Autodesk Fusion 360 part; units mm, degrees
sketch "Sketch1" plane through (0, 0, 0) normal (0, 0, 1) x (1, 0, 0)
  line L0 (0, 0) -> (-27, 0)
  line L1 (-27, 0) -> (-27, 4)
  line L2 (-27, 4) -> (-20.5209, 4)
  line L3 (-20.5209, 4) -> (-20.5209, 6)
  line L4 (-20.5209, 6) -> (-16, 6)
  line L5 (-16, 6) -> (-15, 8)
  line L6 (-15, 8) -> (-11.4968, 8)
  arc A0 (-11.4968, 8) -> (-6, 10) centre (-11.4968, 16.5538) ccw
  line L7 (-6, 10) -> (0, 10)
  line L8 (0, 10) -> (0, 0)
  dimension "d1" = 4
  dimension "d2" = 27
revolve "Revolve1" add sketch "Sketch1" angle 360 about axis through (0, 0, 0) along (-1, 0, 0)
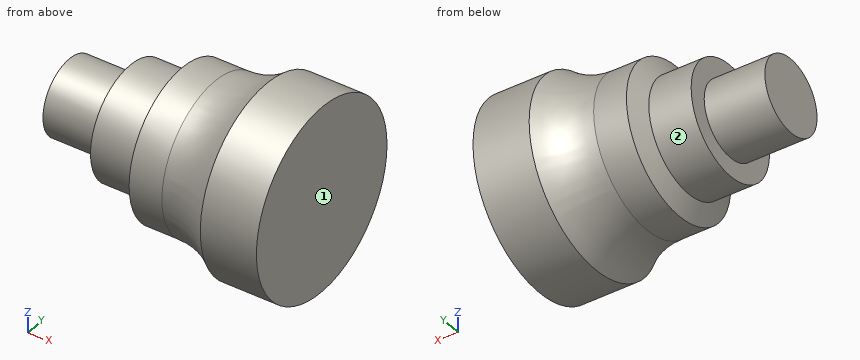
CAD build for the part. Positions are in the model's coordinates, mm. Face numbers are marked on the shaded views. A direction names the side the tool comes from. Give positions to 0.01 mm unless a question says otherwise; leave off trailing zeros. Write each loop counter-clockwise with the first axis right and the second up, starting at its lowest first coordinate (ties: lowest second). Pieces come first, ordered by that corner, then holes. Notation, with made-up numbers: (-20.5, 36.5) - (13.5, 36.5) arc R26 cw to (13.5, 54.5) - close; hole circle Ø8 at (-6, -15.75). An arc over 180 degrees is marked (long way). Put each result on its own line as item: value.
(1) Tool access for the marked faces 1 and 2: list every direction of +Z, -Z, +X, -X, +Y, -Y with a clear straight run to the whole face (end or side of a thin tool).
Working result:
face 1: +Z, -Z, +X, +Y, -Y
face 2: -X
(2) Saw through at C-C (x = -18). List the corners of the cut face in (y, z).
Working result:
outline: circle Ø12 at (0, 0)
(3) Saw through at A-A (z = 0). List the corners of the cut face in (x, y), then the cut area to 3 significant figures.
Working result:
outline: (-27, -4) - (-20.52, -4) - (-20.52, -6) - (-16, -6) - (-15, -8) - (-11.5, -8) arc R8.55 cw to (-6, -10) - (0, -10) - (0, 10) - (-6, 10) arc R8.55 cw to (-11.5, 8) - (-15, 8) - (-16, 6) - (-20.52, 6) - (-20.52, 4) - (-27, 4) - close
area: 391 mm^2
(4) Drop flat-ended pins along their axis: pin 1 Ø2 at (y, z) = (2.5, 7) entering from -X; pin 2 Ø4 at (y, z) = (-6.5, 6) entering from -X; pin 3 Ø4 at (x, z) = (-5, -3) entering from +Y. Give the stop position or say it passes through.
Working result:
pin 1: x = -15.78
pin 2: x = -15.58
pin 3: y = 9.95
(5) Saw through at D-D (x = -12.5). List the corners of the cut face in (y, z).
Working result:
outline: circle Ø16 at (0, 0)
(6) Wall check: L1, parallel to X at y = 3.5, z = -4.5; L2, parallel to Z at x = -21.5, y = 0.25. Give the ranges that are in metal, low to high.
Working result:
L1: -20.52 to 0
L2: -3.99 to 3.99
